from build123d import *

# Parameters (mm, degrees)
BOSS_EXTRUDE1_DEPTH = 3.18
SKETCH2_R           = 1.91
CUT_EXTRUDE4_DEPTH  = 77.192270605


with BuildPart() as part:
    # Sketch1 → Boss-Extrude1 (new body)
    with BuildSketch(Plane(origin=(0, 0, 0), x_dir=(0, 0, -1), z_dir=(1, 0, 0))):
        with BuildLine():
            Line((0, 0), (-67.31, 0))
            Line((-67.31, 0), (-67.31, 33.65))
            ThreePointArc((-67.31, 33.65), (-66.750573952, 35.000573952), (-65.4, 35.56))
            Line((-65.4, 35.56), (0, 35.56))
            Line((0, 35.56), (0, 0))
        make_face()
    extrude(amount=BOSS_EXTRUDE1_DEPTH)

    # Sketch2 → Cut-Extrude4 (cut, through all)
    with BuildSketch(Plane(origin=(3.18, 0, 0), x_dir=(0, 0, -1), z_dir=(1, 0, 0))):
        with Locations((-63.5, 26.67)):
            Circle(SKETCH2_R)
        with Locations((-63.5, 6.35)):
            Circle(SKETCH2_R)
        with Locations((-3.81, 6.35)):
            Circle(SKETCH2_R)
        with Locations((-3.81, 26.67)):
            Circle(SKETCH2_R)
    extrude(amount=-CUT_EXTRUDE4_DEPTH, mode=Mode.SUBTRACT)


solid = part.part
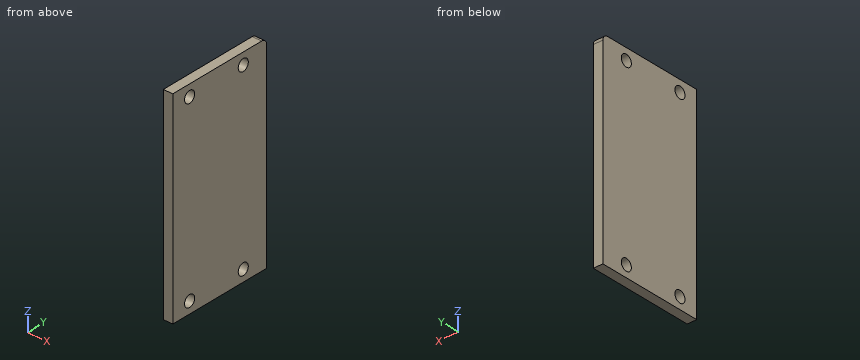
Input: part model. Units: mm. Frame: model coordinates. Give positions to 0.01 mm unless a question says otherwise; leave off trailing zeros. Order: outer loops, then holes, each group sorted by start corner. A loop starts at its lowest first (then second) coordinate and runs counter-clockwise, first axis right, second up. Notation, with made-up numbers: (-37.5, -9.75) -> (-29.5, -9.75) arc R30 ccw to (-29.5, 25.25) -> close; hole circle Ø10 at (-9, 69). An arc over 180 degrees is marked (long way). Use one line per item in the form item = value.
1) Line query: probe 1 along Y at (x, z) = (1.2, 3.81); probe 2 along Z at (x, y) = (0.65, 25); probe 3 along Y at (x, z) = (1.35, 3.5). Output: solid intervals per line, ascending.
Response values:
probe_1 = 0 to 4.44, 8.26 to 24.76, 28.58 to 35.56
probe_2 = 0 to 2.88, 4.74 to 62.57, 64.43 to 67.31
probe_3 = 0 to 4.47, 8.23 to 24.79, 28.55 to 35.56
2) First-contact query: pin 1 Ø1.5 at (y, z) = (10.5, 55) entering from -X. Flat tip, straight axial feed; report the tip coordinate or a pass-through.
Response values:
pin_1 = 0
3) Section B-B, the plane z = 63.5. Return loops of the section in (x, y).
Response values:
outline = (0, 0) -> (3.18, 0) -> (3.18, 4.44) -> (0, 4.44) -> close; (0, 8.26) -> (3.18, 8.26) -> (3.18, 24.76) -> (0, 24.76) -> close; (0, 28.58) -> (3.18, 28.58) -> (3.18, 35.56) -> (0, 35.56) -> close
4) Section A-A, the plane y = 6.35. Return loops of the section in (x, z), and give its area (3 significant figures).
Response values:
outline = (0, 0) -> (3.18, 0) -> (3.18, 1.9) -> (0, 1.9) -> close; (0, 5.72) -> (3.18, 5.72) -> (3.18, 61.59) -> (0, 61.59) -> close; (0, 65.41) -> (3.18, 65.41) -> (3.18, 67.31) -> (0, 67.31) -> close
area = 190 mm^2
5) Section C-C, the plane x = 0.8. Return loops of the section in (y, z), and give its area (3 significant figures).
Response values:
outline = (0, 0) -> (35.56, 0) -> (35.56, 65.4) arc R1.91 ccw to (33.65, 67.31) -> (0, 67.31) -> close; hole circle Ø3.82 at (6.35, 3.81); hole circle Ø3.82 at (6.35, 63.5); hole circle Ø3.82 at (26.67, 3.81); hole circle Ø3.82 at (26.67, 63.5)
area = 2,350 mm^2
